from build123d import *

# Parameters (mm, degrees)
SKETCH1_R          = 1.35
EXTRUDE1_DEPTH     = 23
SKETCH2_R          = 1.35
CUT_EXTRUDE1_DEPTH = 10
CHAMFER3_SIZE      = 1
EXTRUDE2_DEPTH     = 18
EXTRUDE3_DEPTH     = 18


with BuildPart() as part:
    # Sketch1 → Extrude1 (new body)
    with BuildSketch(Plane.XY):
        with BuildLine():
            Line((134.244131426, -107.376468954), (135.270230766, -172.368369374))
            Line((135.270230766, -172.368369374), (107.273719816, -172.810381397))
            Line((107.273719816, -172.810381397), (106.44776294, -120.495264366))
            ThreePointArc((106.44776294, -120.495264366), (116.078507859, -115.825445612), (122.873690334, -107.555986741))
            Line((122.873690334, -107.555986741), (134.244131426, -107.376468954))
        make_face()
        with Locations((110.720688645, -137.750476655)):
            Circle(SKETCH1_R, mode=Mode.SUBTRACT)
        with Locations((111.178504518, -166.747984476)):
            Circle(SKETCH1_R, mode=Mode.SUBTRACT)
        with Locations((124.176884602, -166.542764608)):
            Circle(SKETCH1_R, mode=Mode.SUBTRACT)
        with Locations((123.987450878, -154.544259915)):
            Circle(SKETCH1_R, mode=Mode.SUBTRACT)
        with Locations((110.989070794, -154.749479783)):
            Circle(SKETCH1_R, mode=Mode.SUBTRACT)
        with Locations((123.529652711, -125.547873574)):
            Circle(SKETCH1_R, mode=Mode.SUBTRACT)
        with Locations((110.531272627, -125.753093442)):
            Circle(SKETCH1_R, mode=Mode.SUBTRACT)
        with Locations((123.340218986, -113.549368881)):
            Circle(SKETCH1_R, mode=Mode.SUBTRACT)
        with Locations((128.65529324, -133.466326068)):
            Circle(SKETCH1_R, mode=Mode.SUBTRACT)
        with Locations((110.862781644, -146.750476655)):
            Circle(SKETCH1_R, mode=Mode.SUBTRACT)
        with Locations((128.860538683, -146.466326068)):
            Circle(SKETCH1_R, mode=Mode.SUBTRACT)
    extrude(amount=EXTRUDE1_DEPTH)

    # Sketch2 → Cut-Extrude1 (cut)
    with BuildSketch(Plane(origin=(132.515828327, 2.092174611, 0), x_dir=(0, 0, -1), z_dir=(0.9998753910699589, 0.01578614369301875, 0))):
        with Locations(Location((-16, -114.482286036, 0), (0, 0, 90))):
            Circle(SKETCH2_R)
        with Locations(Location((-4, -114.482286036, 0), (0, 0, 90))):
            Circle(SKETCH2_R)
        with Locations(Location((-16, -124.482286036, 0), (0, 0, 90))):
            Circle(SKETCH2_R)
        with Locations(Location((-4, -124.482286036, 0), (0, 0, 90))):
            Circle(SKETCH2_R)
        with Locations(Location((-16, -169.482286036, 0), (0, 0, 90))):
            Circle(SKETCH2_R)
        with Locations(Location((-4, -169.482286036, 0), (0, 0, 90))):
            Circle(SKETCH2_R)
        with Locations(Location((-16, -159.482286036, 0), (0, 0, 90))):
            Circle(SKETCH2_R)
        with Locations(Location((-4, -159.482286036, 0), (0, 0, 90))):
            Circle(SKETCH2_R)
    extrude(amount=-CUT_EXTRUDE1_DEPTH, mode=Mode.SUBTRACT)

    # Chamfer3
    # the kernel refuses this chamfer: 1 mm, written as the material it takes off along each edge
    with BuildSketch(Plane(origin=(107.273719816, -172.810381397, -2.571682988), x_dir=(-0.01578614369302038, 0.9998753910699589, 0), z_dir=(0, 0, 1))) as chamfer3_piece_1:
        Polygon((CHAMFER3_SIZE, 0), (0, -CHAMFER3_SIZE), (0, 0), align=None)
    extrude(amount=28.143365976, mode=Mode.SUBTRACT)
    with BuildSketch(Plane(origin=(106.44776294, -120.495264366, -2.646322056), x_dir=(0.9673390331642948, 0.2534860842665082, 0), z_dir=(0, 0, 1))) as chamfer3_piece_2:
        with BuildLine():
            Line((1.026523691, 0), (-CHAMFER3_SIZE * 0.238183944659, -CHAMFER3_SIZE * 0.971220061833))
            Line((-CHAMFER3_SIZE * 0.238183944659, -CHAMFER3_SIZE * 0.971220061833), (0, 0))
            ThreePointArc((0, 0), (0.529135289, -0.00526427), (1.026523691, 0))
        make_face()
    extrude(amount=28.292644112, mode=Mode.SUBTRACT)
    with BuildSketch(Plane(origin=(122.873690334, -107.555986741, -2.676981296), x_dir=(0.9998753910699592, 0.015786143693006172, 0), z_dir=(0, 0, 1))) as chamfer3_piece_3:
        with BuildLine():
            Line((CHAMFER3_SIZE, 0), (-0.504457815, -0.904781971))
            ThreePointArc((-0.504457815, -0.904781971), (-0.256001011, -0.470163527), (0, 0))
            Line((0, 0), (CHAMFER3_SIZE, 0))
        make_face()
    extrude(amount=28.353962591, mode=Mode.SUBTRACT)

    # Sketch3 → Extrude2 (cut)
    with BuildSketch(Plane.XY.offset(23)):
        with BuildLine():
            Line((104.011515413, -130.855030895), (131.107623287, -130.427234536))
            ThreePointArc((131.107623287, -130.427234536), (132.175086772, -130.849775884), (132.631115589, -131.903368407))
            Line((132.631115589, -131.903368407), (132.883719463, -147.90299458))
            ThreePointArc((132.883719463, -147.90299458), (132.461178115, -148.970458066), (131.407585592, -149.426486882))
            Line((131.407585592, -149.426486882), (104.311477719, -149.854283242))
            ThreePointArc((104.311477719, -149.854283242), (103.244014233, -149.431741893), (102.787985417, -148.378149371))
            Line((102.787985417, -148.378149371), (102.535381542, -132.378523198))
            ThreePointArc((102.535381542, -132.378523198), (102.957922891, -131.311059712), (104.011515413, -130.855030895))
        make_face()
    extrude(amount=-EXTRUDE2_DEPTH, mode=Mode.SUBTRACT)

    # Sketch4 → Extrude3 (cut)
    with BuildSketch(Plane(origin=(0, 0, 0), x_dir=(-1, 0, 0), z_dir=(0, 0, -1))):
        with BuildLine():
            Line((-128.995288436, -91.654520496), (-129.552584273, -126.952969799))
            ThreePointArc((-129.552584273, -126.952969799), (-129.130042924, -128.020433284), (-128.076450401, -128.476462101))
            Line((-128.076450401, -128.476462101), (-95.502554389, -128.990742388))
            ThreePointArc((-95.502554389, -128.990742388), (-94.435090904, -128.568201039), (-93.979062087, -127.514608517))
            Line((-93.979062087, -127.514608517), (-93.42176625, -92.216159214))
            ThreePointArc((-93.42176625, -92.216159214), (-93.844307599, -91.148695728), (-94.897900122, -90.692666912))
            Line((-94.897900122, -90.692666912), (-127.471796134, -90.178386625))
            ThreePointArc((-127.471796134, -90.178386625), (-128.539259619, -90.600927973), (-128.995288436, -91.654520496))
        make_face()
        with BuildLine():
            Line((-129.963024009, -152.949729966), (-130.439103933, -183.104060885))
            ThreePointArc((-130.439103933, -183.104060885), (-130.016562585, -184.17152437), (-128.962970062, -184.627553187))
            Line((-128.962970062, -184.627553187), (-101.681956846, -185.058268853))
            ThreePointArc((-101.681956846, -185.058268853), (-100.61449336, -184.635727504), (-100.158464544, -183.582134982))
            Line((-100.158464544, -183.582134982), (-99.682384619, -153.427804063))
            ThreePointArc((-99.682384619, -153.427804063), (-100.104925968, -152.360340578), (-101.15851849, -151.904311761))
            Line((-101.15851849, -151.904311761), (-128.439531706, -151.473596095))
            ThreePointArc((-128.439531706, -151.473596095), (-129.506995192, -151.896137444), (-129.963024009, -152.949729966))
        make_face()
    extrude(amount=-EXTRUDE3_DEPTH, mode=Mode.SUBTRACT)


solid = part.part
The model under review builds one solid part; all positions refer to its coordinate system, in mm. A direction names the side the tool comes from. Round coordinates to 2 decimals unless told otherwise and drop trailing zeros. Loops run counter-clockwise (first coordinate to the right, second up) from the corner with the lowest first, then second, coordinate; pieces in that order, holes last. Notation, with made-up numbers: (56, -2.5) -> (103, -2.5) arc R20 ccw to (103, 4.5) -> close; hole circle Ø8 at (2, -29). An arc over 180 degrees is marked (long way). Return JSON: item names as keys, results as strings.
(1) For line 1 (Y direction, x = 122.5, z = 20); line 2 (Z direction, x = 118.25, y = -160.5); line 3 (X direction, y = -126.5, z = 19), list the stretches that pass through material, from the lowest coordinate up.
Solved:
{"line 1": "-172.57 to -149.57, -130.56 to -126.42, -124.67 to -114.61, -112.49 to -108.4", "line 2": "18 to 23", "line 3": "106.54 to 109.41, 111.66 to 122.57, 124.49 to 134.55"}
(2) For faces 4 (the cylindrical face through (111.82, -125.35, 20.46)), 5 (the cylindrical face through (132.163, -130.838, 14.126)), 6 (the cylindrical face through (132.548, -156.122, 16.406)), list the 3-axis set-ups (+Z, -Z, +X, -X, +Y, -Y) from which the entire face can be reached by the end or side of a thin tool; tool diameter is ignored.
Solved:
{"face 4": "+Z, -Z", "face 5": "+Z", "face 6": "none"}
(3) Add section C-C on z = 19.25. Write out the cut boundary in (x, y).
Solved:
{"outline": "(106.46, -121.5) -> (106.61, -130.81) -> (131.11, -130.43) arc R1.5 cw to (132.63, -131.9) -> (132.88, -147.9) arc R1.5 cw to (131.41, -149.43) -> (106.91, -149.81) -> (107.26, -171.81) -> (108.27, -172.79) -> (135.27, -172.37) -> (134.24, -107.38) -> (123.87, -107.54) -> (122.38, -108.47) arc R25 cw to (107.44, -120.24) -> close; hole circle Ø2.7 at (110.53, -125.75); hole circle Ø2.7 at (110.99, -154.75); hole circle Ø2.7 at (111.18, -166.75); hole circle Ø2.7 at (123.34, -113.55); hole circle Ø2.7 at (123.53, -125.55); hole circle Ø2.7 at (123.99, -154.54); hole circle Ø2.7 at (124.18, -166.54)"}
(4) Add section D-D on x = 114.75. Write out the cut boundary in (y, z), plus the area to 3 significant figures.
Solved:
{"outline": "(-172.69, 18) -> (-151.69, 18) -> (-151.69, 0) -> (-128.69, 0) -> (-128.69, 18) -> (-116.8, 18) -> (-116.8, 23) -> (-130.69, 23) -> (-130.69, 5) -> (-149.69, 5) -> (-149.69, 23) -> (-172.69, 23) -> close", "area": "351 mm2"}
(5) Add section A-A on x = 111.25. State how many separate pieces and enclosed holes the cut face has, plus the area to 3 significant figures.
Solved:
{"separate pieces": "6", "enclosed holes": "0", "area": "278 mm2"}
(6) Add section B-B on z = 12. Write out the cut boundary in (x, y).
Solved:
{"outline": "(106.58, -128.82) -> (106.61, -130.81) -> (131.11, -130.43) arc R1.5 cw to (132.63, -131.9) -> (132.88, -147.9) arc R1.5 cw to (131.41, -149.43) -> (106.91, -149.81) -> (106.94, -151.81) -> (128.44, -151.47) arc R1.5 cw to (129.96, -152.95) -> (130.27, -172.45) -> (135.27, -172.37) -> (134.24, -107.38) -> (129.24, -107.46) -> (129.55, -126.95) arc R1.5 cw to (128.08, -128.48) -> close"}
(7) For pin 1 (12 mm diameter, centred on x = 127, z = 5.5, fed in from -Y); pin 2 (8 mm diameter, centred on y = -134, z = 17, fed in from -X); pin 3 (2 mm diameter, centred on x = 117, z = 11.5, fed in from -Y); pin 4 (2 mm diameter, centred on x = 111.18, y = -166.75, fed in from +Z), all flat-tipped, find the tip position at first contact; note any pin that passes through.
Solved:
{"pin 1": "y = -172.45", "pin 2": "x = 106.6", "pin 3": "y = -151.67", "pin 4": "through"}
(8) The part is to be moulded in two halves that separate along X. For faces 1 (the flat face through (121, -120, 18)), 2 (the flat face through (106.959, -120.856, 20.465)), 3 (the cylindrical face through (112.008, -137.345, 2.465)), say which applies: released by +X, released by -X, zero draft, split by the parting line, or undercut.
Solved:
{"face 1": "zero draft", "face 2": "released by -X", "face 3": "undercut"}
